```python
from build123d import *

# Parameters (mm, degrees)
F1_DEPTH = 25.4
F2_R     = 9.525
F3_DEPTH = 25.4


# Not quite as in the source:
# - a pattern or mirror of a feature is missing from the dataset's text; its kind, count and spacing are read off the source's solid


with BuildPart() as f1:
    # F0 (on Front) → F1 (new body)
    with BuildSketch(Plane.XZ):
        with BuildLine():
            Line((38.1, 53.975), (-38.1, 53.975))
            Line((-38.1, 53.975), (-38.1, -15.875))
            Line((-38.1, -15.875), (12.7, -15.875))
            ThreePointArc((12.7, -15.875), (19.05, -22.225), (12.7, -28.575))
            Line((12.7, -28.575), (-38.1, -28.575))
            Line((-38.1, -28.575), (-38.1, -53.975))
            Line((-38.1, -53.975), (38.1, -53.975))
            Line((38.1, -53.975), (38.1, 15.875))
            Line((38.1, 15.875), (-12.7, 15.875))
            ThreePointArc((-12.7, 15.875), (-19.05, 22.225), (-12.7, 28.575))
            Line((-12.7, 28.575), (38.1, 28.575))
            Line((38.1, 28.575), (38.1, 53.975))
        make_face()
    extrude(amount=F1_DEPTH)

    # F2 (on face) → F3 (cut, through all)
    with BuildSketch(Plane.XY.offset(53.975)):
        with Locations((0, -12.7)):
            Circle(F2_R)
    f3 = extrude(amount=-F3_DEPTH, mode=Mode.SUBTRACT)

    # F3_copies: F3 across plane
    add(f3.mirror(Plane(origin=(0, 0, 0), x_dir=(-1, 0, 0), z_dir=(0, 0, -1))), mode=Mode.SUBTRACT)


solid = f1.part
```
For this review, take the finished solid that the model builds, in its own axes (mm). A direction names the side the tool comes from. Coordinates: 2 decimals unless noted, no trailing zeros. Write each loop counter-clockwise with the first axis right and the second up, starting at its lowest first coordinate (ties: lowest second). Pieces come first, ordered by that corner, then holes.
(1) Add section D-D on z = 41.5. Give the boundary of the cut face in (x, y) (3 decimals).
(2) The part is to be moulded in two halves that separate along X. For faces 1 (the face through (19.05, -12.52, -22.09)), 2 (the face through (8, -7, -53.975)), 3 (the face through (-1.24, -3.256, 41.453)), 4 (the face through (38.1, -13, 41)), say which applies: +X half, -X half, draft (parallel to the pull), parting line (faces both ways), or undercut.
(3) Add section C-C on x = 0. Give the boundary of the cut face in (y, z) (3 decimals).
(4) Add section B-B on y = -12.7. Give the boundary of the cut face in (x, z) (3 decimals).
(5) Tool access review of faces 5 (the face through (-18, -13, -28.575)), 6 (the face through (-1.24, -3.256, -41.453)), 7 (the face through (18, -13, 28.575)), 8 (the face through (-1, 0, 1)), 9 (the face through (-38.1, -13, -41)): name each direction out of +Z, -Z, +X, -X, +Y, -Y from which nothing blocks a thin tool from reaching the whole face with its end or side.
(6) Wall thickness on probe 1 along Z at (x, y) = (-13, -8.25) (3 decimals); probe 2 along Y at (x, z) = (0, -48) (3 decimals); probe 3 along Z at (x, y) = (27, -10.75) (3 decimals): over which ranges is each line inside the solid? List them lowest first.
(7) Add section A-A on x = -33. Give the boundary of the cut face in (y, z) (3 decimals).
Answer sheet:
1. outline: (-38.1, -25.4) - (38.1, -25.4) - (38.1, 0) - (-38.1, 0) - close; hole circle Ø19.05 at (0, -12.7)
2. face 1: -X half
2. face 2: draft
2. face 3: undercut
2. face 4: +X half
3. outline: (-25.4, -53.975) - (-22.225, -53.975) - (-22.225, -28.575) - (-25.4, -28.575) - close; (-25.4, -15.875) - (0, -15.875) - (0, 15.875) - (-25.4, 15.875) - close; (-25.4, 28.575) - (-22.225, 28.575) - (-22.225, 53.975) - (-25.4, 53.975) - close; (-3.175, -53.975) - (0, -53.975) - (0, -28.575) - (-3.175, -28.575) - close; (-3.175, 28.575) - (0, 28.575) - (0, 53.975) - (-3.175, 53.975) - close
4. outline: (-38.1, -53.975) - (-9.525, -53.975) - (-9.525, -28.575) - (-38.1, -28.575) - close; (-38.1, -15.875) - (12.7, -15.875) arc R6.35 cw to (12.7, -28.575) - (9.525, -28.575) - (9.525, -53.975) - (38.1, -53.975) - (38.1, 15.875) - (-12.7, 15.875) arc R6.35 cw to (-12.7, 28.575) - (-9.525, 28.575) - (-9.525, 53.975) - (-38.1, 53.975) - close; (9.525, 28.575) - (38.1, 28.575) - (38.1, 53.975) - (9.525, 53.975) - close
5. face 5: -X, +Y, -Y
5. face 6: -Z
5. face 7: +X, +Y, -Y
5. face 8: +Z, -Z, +X, -X, +Y
5. face 9: +Z, -Z, -X, +Y, -Y
6. probe 1: z = -53.975 to -28.575, -15.875 to 15.882, 28.568 to 53.975
6. probe 2: y = -25.4 to -22.225, -3.175 to 0
6. probe 3: z = -53.975 to 15.875, 28.575 to 53.975
7. outline: (-25.4, -53.975) - (0, -53.975) - (0, -28.575) - (-25.4, -28.575) - close; (-25.4, -15.875) - (0, -15.875) - (0, 53.975) - (-25.4, 53.975) - close
